Could you check a few things on this model? Use its own coordinates, in mm. A direction names the side the tool comes from. Give positions to 0.01 mm unless a question says otherwise; leave off trailing zeros. Write item = value, one per line.
from build123d import *

# Parameters (mm, degrees)
SKETCH1_W            = 260.35
SKETCH1_H            = 16.51
BOSS_EXTRUDE1_DEPTH  = 254
SKETCH2_W            = 33.655
SKETCH2_H            = 9.144
CUT_EXTRUDE1_DEPTH   = 286.534018376
LPATTERN1_COUNT      = 7
LPATTERN1_PITCH      = 35.56
SKETCH3_R            = 12.065
CUT_EXTRUDE2_DEPTH   = 286.891781493
LPATTERN2_COUNT      = 7
LPATTERN2_PITCH      = 35.56
LPATTERN2_COUNT_DIR2 = 8
LPATTERN2_PITCH_DIR2 = 30.734


with BuildPart() as part:
    # Sketch1 → Boss-Extrude1 (new body)
    with BuildSketch(Plane(origin=(0, 0, 0), x_dir=(1, 0, 0), z_dir=(0, 1, 0))):
        Rectangle(SKETCH1_W, SKETCH1_H)
    extrude(amount=BOSS_EXTRUDE1_DEPTH)

    # Sketch2 → Cut-Extrude1 (cut, through all)
    with BuildSketch(Plane(origin=(0, 254, 0), x_dir=(1, 0, 0), z_dir=(0, 1, 0))):
        with Locations((-108.1405, 0)):
            Rectangle(SKETCH2_W, SKETCH2_H)
    cut_extrude1 = extrude(amount=-CUT_EXTRUDE1_DEPTH, mode=Mode.SUBTRACT)

    # LPattern1: Cut-Extrude1 ×7
    with Locations(*[(i * LPATTERN1_PITCH, 0, 0) for i in range(1, LPATTERN1_COUNT)]):
        add(cut_extrude1, mode=Mode.SUBTRACT)

    # Sketch3 → Cut-Extrude2 (cut, through all)
    with BuildSketch(Plane.XY.offset(8.255)):
        with Locations((-108.585, 233.68)):
            Circle(SKETCH3_R)
    cut_extrude2 = extrude(amount=-CUT_EXTRUDE2_DEPTH, mode=Mode.SUBTRACT)

    # LPattern2: Cut-Extrude2 7 × 8
    with Locations(*[(i * LPATTERN2_PITCH, -j * LPATTERN2_PITCH_DIR2, 0) for i in range(LPATTERN2_COUNT) for j in range(LPATTERN2_COUNT_DIR2) if (i, j) != (0, 0)]):
        add(cut_extrude2, mode=Mode.SUBTRACT)


solid = part.part
1. I need wall thicknesses on line 1 (Z direction, x = 114, y = 153) (3 decimals). Which ranges of the line are inside material? Lowest first, please.
Filled sheet:
line_1 = -8.255 to -4.572, 4.572 to 8.255
2. For pin 1 (21.5 mm diameter, centred on x = -37.465, y = 233.68, fed in from -Z), with a flat end and sliding along its axis, tell me the tip position at first contact or that it passes through.
Filled sheet:
pin_1 = through
3. Thinking about a two-plate mould opening in Y: for faces 1 (the face through (88.392, 129, 0)), 2 (the face through (-2, 0, -6)), 3 (the face through (-74.6, 91.97, -6.39)), which applies, pulls with the +Y half, pulls with the -Y half, needs draft (parallel to the pull), parting line crosses it, or undercut?
Filled sheet:
face_1 = needs draft
face_2 = pulls with the -Y half
face_3 = undercut
4. If we section it at A-A, the plane z = 0.75: Count the separate pieces of the cut face and the enclosed holes in it, and give its area (3 significant figures).
Filled sheet:
separate_pieces = 8
enclosed_holes = 0
area = 6,290 mm2
5. Which directions (+Z, -Z, +X, -X, +Y, -Y) give clear straight access to the entire face, cutting with the end or side of a thin tool? Please do faces 4 (the face through (66.6, 129.7, 6.4)), 5 (the face through (-124.968, 129, 0)).
Filled sheet:
face_4 = +Z, -Z
face_5 = +Y, -Y
